Autodesk Inventor part; units mm, degrees
ref_plane "YZ Plane" through (0, 0, 0) normal (1, 0, 0) x (0, 1, 0)
ref_plane "XZ Plane" through (0, 0, 0) normal (0, 1, 0) x (-1, 0, 0)
ref_plane "XY Plane" through (0, 0, 0) normal (0, 0, 1) x (1, 0, 0)
sketch "Sketch2" plane through (0, 0, 0) normal (1, 0, 0) x (0, 1, 0)
  circle A0 centre (0, 0) radius 15 construction
  circle A1 centre (0, 0) radius 18 construction
  line L0 (17.7784, 2.8158) -> (17.7784, -2.8158) construction
  line L1 (17.7784, 2.8158) -> (0, 0) construction
  line L2 (0, 0) -> (17.7784, -2.8158) construction
  line L3 (17.7784, 2.8158) -> (19.9784, 0)
  line L4 (19.9784, 0) -> (17.7784, -2.8158)
  line L5 (19.9784, 0) -> (17.7784, 0) construction
  line L6 (14.8153, 2.3465) -> (13.8153, 0)
  line L7 (13.8153, 0) -> (14.8153, -2.3465)
  line L8 (14.8153, 2.3465) -> (14.8153, -2.3465) construction
  line L9 (13.8153, 0) -> (14.8153, 0) construction
  line L10 (16.0381, 8.1718) -> (19.0006, 6.1737)
  line L11 (19.0006, 6.1737) -> (17.7784, 2.8158)
  line L12 (13.3651, 6.8099) -> (13.1392, 4.2692)
  line L13 (13.1392, 4.2692) -> (14.8153, 2.3465)
  line L14 (12.7279, 12.7279) -> (16.1629, 11.743)
  line L15 (16.1629, 11.743) -> (16.0381, 8.1718)
  line L16 (10.6066, 10.6066) -> (11.1768, 8.1204)
  line L17 (11.1768, 8.1204) -> (13.3651, 6.8099)
  line L18 (8.1718, 16.0381) -> (11.743, 16.1629)
  line L19 (11.743, 16.1629) -> (12.7279, 12.7279)
  line L20 (6.8099, 13.3651) -> (8.1204, 11.1768)
  line L21 (8.1204, 11.1768) -> (10.6066, 10.6066)
  line L22 (2.8158, 17.7784) -> (6.1737, 19.0006)
  line L23 (6.1737, 19.0006) -> (8.1718, 16.0381)
  line L24 (2.3465, 14.8153) -> (4.2692, 13.1392)
  line L25 (4.2692, 13.1392) -> (6.8099, 13.3651)
  line L26 (-2.8158, 17.7784) -> (0, 19.9784)
  line L27 (0, 19.9784) -> (2.8158, 17.7784)
  line L28 (-2.3465, 14.8153) -> (0, 13.8153)
  line L29 (0, 13.8153) -> (2.3465, 14.8153)
  line L30 (-8.1718, 16.0381) -> (-6.1737, 19.0006)
  line L31 (-6.1737, 19.0006) -> (-2.8158, 17.7784)
  line L32 (-6.8099, 13.3651) -> (-4.2692, 13.1392)
  line L33 (-4.2692, 13.1392) -> (-2.3465, 14.8153)
  line L34 (-12.7279, 12.7279) -> (-11.743, 16.1629)
  line L35 (-11.743, 16.1629) -> (-8.1718, 16.0381)
  line L36 (-10.6066, 10.6066) -> (-8.1204, 11.1768)
  line L37 (-8.1204, 11.1768) -> (-6.8099, 13.3651)
  line L38 (-16.0381, 8.1718) -> (-16.1629, 11.743)
  line L39 (-16.1629, 11.743) -> (-12.7279, 12.7279)
  line L40 (-13.3651, 6.8099) -> (-11.1768, 8.1204)
  line L41 (-11.1768, 8.1204) -> (-10.6066, 10.6066)
  line L42 (-17.7784, 2.8158) -> (-19.0006, 6.1737)
  line L43 (-19.0006, 6.1737) -> (-16.0381, 8.1718)
  line L44 (-14.8153, 2.3465) -> (-13.1392, 4.2692)
  line L45 (-13.1392, 4.2692) -> (-13.3651, 6.8099)
  line L46 (-17.7784, -2.8158) -> (-19.9784, 0)
  line L47 (-19.9784, 0) -> (-17.7784, 2.8158)
  line L48 (-14.8153, -2.3465) -> (-13.8153, 0)
  line L49 (-13.8153, 0) -> (-14.8153, 2.3465)
  line L50 (-16.0381, -8.1718) -> (-19.0006, -6.1737)
  line L51 (-19.0006, -6.1737) -> (-17.7784, -2.8158)
  line L52 (-13.3651, -6.8099) -> (-13.1392, -4.2692)
  line L53 (-13.1392, -4.2692) -> (-14.8153, -2.3465)
  line L54 (-12.7279, -12.7279) -> (-16.1629, -11.743)
  line L55 (-16.1629, -11.743) -> (-16.0381, -8.1718)
  line L56 (-10.6066, -10.6066) -> (-11.1768, -8.1204)
  line L57 (-11.1768, -8.1204) -> (-13.3651, -6.8099)
  line L58 (-8.1718, -16.0381) -> (-11.743, -16.1629)
  line L59 (-11.743, -16.1629) -> (-12.7279, -12.7279)
  line L60 (-6.8099, -13.3651) -> (-8.1204, -11.1768)
  line L61 (-8.1204, -11.1768) -> (-10.6066, -10.6066)
  line L62 (-2.8158, -17.7784) -> (-6.1737, -19.0006)
  line L63 (-6.1737, -19.0006) -> (-8.1718, -16.0381)
  line L64 (-2.3465, -14.8153) -> (-4.2692, -13.1392)
  line L65 (-4.2692, -13.1392) -> (-6.8099, -13.3651)
  line L66 (2.8158, -17.7784) -> (0, -19.9784)
  line L67 (0, -19.9784) -> (-2.8158, -17.7784)
  line L68 (2.3465, -14.8153) -> (0, -13.8153)
  line L69 (0, -13.8153) -> (-2.3465, -14.8153)
  line L70 (8.1718, -16.0381) -> (6.1737, -19.0006)
  line L71 (6.1737, -19.0006) -> (2.8158, -17.7784)
  line L72 (6.8099, -13.3651) -> (4.2692, -13.1392)
  line L73 (4.2692, -13.1392) -> (2.3465, -14.8153)
  line L74 (12.7279, -12.7279) -> (11.743, -16.1629)
  line L75 (11.743, -16.1629) -> (8.1718, -16.0381)
  line L76 (10.6066, -10.6066) -> (8.1204, -11.1768)
  line L77 (8.1204, -11.1768) -> (6.8099, -13.3651)
  line L78 (16.0381, -8.1718) -> (16.1629, -11.743)
  line L79 (16.1629, -11.743) -> (12.7279, -12.7279)
  line L80 (13.3651, -6.8099) -> (11.1768, -8.1204)
  line L81 (11.1768, -8.1204) -> (10.6066, -10.6066)
  line L82 (17.7784, -2.8158) -> (19.0006, -6.1737)
  line L83 (19.0006, -6.1737) -> (16.0381, -8.1718)
  line L84 (14.8153, -2.3465) -> (13.1392, -4.2692)
  line L85 (13.1392, -4.2692) -> (13.3651, -6.8099)
  dimension "d15" = 30
  dimension "d16" = 36
  dimension "d19" = 18
  dimension "d20" = 2.2
  dimension "d22" = 1
  dimension "d25" = 360
extrude "Extrusion2" add sketch "Sketch2" along normal blind 60
properties part number "FlexRoller" material "PC/ABS Plastic"
Build history of the part. All positions in model axes, mm. A direction names the side the tool comes from. Round coordinates to 2 decimals unless told otherwise and drop trailing zeros. Order: outer loops, then holes, each group sorted by start corner. A loop starts at its lowest first (then second) coordinate and runs counter-clockwise, first axis right, second up. Notation, with made-up numbers: (51, -14) - (67, -14) arc R27 cw to (67, 13) - close; hole circle Ø7 at (49, 65.25). An arc over 180 degrees is marked (long way). Use a Markdown table: item, result.
1) Pull direction Y, two halves, no side cores. Call faces 5 (the face through (29.58, 18.4, 4.52)), 6 (the face through (29.58, 1.16, 14.31)), 7 (the face through (29.58, -18.38, 4.47)): pulls with the +Y half, pulls with the -Y half, needs draft (parallel to the pull), parting line crosses it, or undercut.
Recorded:
| item | result |
|---|---|
| face 5 | pulls with the +Y half |
| face 6 | undercut |
| face 7 | pulls with the -Y half |
2) Tool access for faces 1 (the face through (29.58, -18.89, 1.39)), 2 (the face through (29.58, -3.294, -13.989)), 3 (the face through (29.58, 1.43, -18.86)), 4 (the face through (29.58, -12.23, -14.47)): list every direction of +Z, -Z, +X, -X, +Y, -Y with a clear straight run to the whole face (end or side of a thin tool).
Recorded:
| item | result |
|---|---|
| face 1 | +X, -X, -Y |
| face 2 | +X, -X |
| face 3 | -Z, +X, -X |
| face 4 | -Z, +X, -X, -Y |
3) Wall check: L1, parallel to Z at x = 36, y = -14.5; L2, parallel to Z at x = 26, y = -4; L3, parallel to Y at x = 39.5, z = 2.5. Give the ranges that are in metal, low to high.
Recorded:
| item | result |
|---|---|
| L1 | z = -12.22 to -2.71, -1.61 to 1.61, 2.71 to 12.22 |
| L2 | z = -18.21 to -13.37, 13.37 to 18.21 |
| L3 | y = -18.03 to -14.68, 14.68 to 18.03 |
4) Saw through at B-B on z = 9.5. Write the cut outline in (x, y).
Recorded:
| item | result |
|---|---|
| outline | (0, -16.08) - (60, -16.08) - (60, -10.86) - (0, -10.86) - close; (0, 10.86) - (60, 10.86) - (60, 16.08) - (0, 16.08) - close |
5) Flat gauge pins, fed straight in: pin 1 Ø6 at (x, y) = (41.5, 9.5) entering from +Z; pin 2 Ø10 at (x, z) = (42.5, -15.5) entering from -Y; pin 3 Ø1.5 at (x, z) = (14, 3) entering from +Y. Where does each tip first touch, or does it go through?
Recorded:
| item | result |
|---|---|
| pin 1 | stops at z = 18.52 |
| pin 2 | stops at y = -16.16 |
| pin 3 | stops at y = 18.22 |
6) Saw through at A-A on z = 1. Write the cut outline in (x, y).
Recorded:
| item | result |
|---|---|
| outline | (0, -19.2) - (60, -19.2) - (60, -14.24) - (0, -14.24) - close; (0, 14.24) - (60, 14.24) - (60, 19.2) - (0, 19.2) - close |
